Work out the finished part from the listing and answer in its coordinate system (mm). Give positions to 0.01 mm unless a question says otherwise; leave off trailing zeros. Loops run counter-clockwise (first coordinate to the right, second up) from the corner with the lowest first, then second, coordinate; pieces in that order, holes last. Notation, with made-up numbers: (62, 70) - (89, 70) arc R15 cw to (89, 94) - close; hole circle Ø2 at (-7, 31). An arc over 180 degrees is marked (long way). Use CSV: the item, a comma, the result in double quotes.
from build123d import *

# Parameters (mm, degrees)
F0_W     = 30
F0_H     = 34
F0_R     = 1.5
F1_DEPTH = 22
F2_R     = 3.95
F3_DEPTH = 32.7


with BuildPart() as f1:
    # F0 (on Top) → F1 (new body)
    with BuildSketch(Plane.XY):
        with Locations((-15, 17)):
            Rectangle(F0_W, F0_H)
        with Locations((-24, 5)):
            Circle(F0_R, mode=Mode.SUBTRACT)
        with Locations((-6, 5)):
            Circle(F0_R, mode=Mode.SUBTRACT)
        with Locations((-24, 29)):
            Circle(F0_R, mode=Mode.SUBTRACT)
        with Locations((-6, 29)):
            Circle(F0_R, mode=Mode.SUBTRACT)
    extrude(amount=F1_DEPTH)

    # F2 (on face) → F3 (cut)
    with BuildSketch(Plane.YZ):
        with Locations((17, 11)):
            Circle(F2_R)
    extrude(amount=-F3_DEPTH, mode=Mode.SUBTRACT)


solid = f1.part
Item 1: A cutting plane is placed at B-B on x = -24. Determine the outline of the cut face in (y, z).
Determined:
outline,"(0, 0) - (3.5, 0) - (3.5, 22) - (0, 22) - close; (6.5, 0) - (27.5, 0) - (27.5, 22) - (6.5, 22) - close; (30.5, 0) - (34, 0) - (34, 22) - (30.5, 22) - close; hole circle Ø7.9 at (17, 11)"
Item 2: Given P1, Ø6, axis at y = 21, z = 2.5, coming from the +X side, flat-ended and moving along its own axis, determine where the tip first touches the part or whether it passes through.
Determined:
P1,"stops at x = 0"
Item 3: A cutting plane is placed at C-C on y = 5. Determine the outline of the cut face in (x, z).
Determined:
outline,"(-30, 0) - (-25.5, 0) - (-25.5, 22) - (-30, 22) - close; (-22.5, 0) - (-7.5, 0) - (-7.5, 22) - (-22.5, 22) - close; (-4.5, 0) - (0, 0) - (0, 22) - (-4.5, 22) - close"
Item 4: The mould has two halves that part along Y. Classify faces 1 (the cylindrical face through (-24.195, 30.487, 10.846)), 2 (the flat face through (-30, 13, 8)), 3 (the flat face through (-15, 34, 11)): pulls with the +Y half, pulls with the -Y half, needs draft (parallel to the pull), parting line crosses it, or undercut.
Determined:
face 1,"undercut"
face 2,"needs draft"
face 3,"pulls with the +Y half"
Item 5: A cutting plane is placed at A-A on z = 11. Determine the outline of the cut face in (x, y), and give its area (3 significant figures).
Determined:
outline,"(-30, 0) - (0, 0) - (0, 13.05) - (-30, 13.05) - close; (-30, 20.95) - (0, 20.95) - (0, 34) - (-30, 34) - close; hole circle Ø3 at (-24, 5); hole circle Ø3 at (-24, 29); hole circle Ø3 at (-6, 5); hole circle Ø3 at (-6, 29)"
area,"755 mm²"
Item 6: Find the intervals of material crossed by line 1 (Y direction, x = -6, z = 12); line 2 (Y direction, x = -18.5, z = 13.5); line 3 (Z direction, x = -19.75, y = 17), in increasing order.
Determined:
line 1,"y = 0 to 3.5, 6.5 to 13.18, 20.82 to 27.5, 30.5 to 34"
line 2,"y = 0 to 13.94, 20.06 to 34"
line 3,"z = 0 to 7.05, 14.95 to 22"
Item 7: A cutting plane is placed at D-D on y = 17. Determine the outline of the cut face in (x, z).
Determined:
outline,"(-30, 0) - (0, 0) - (0, 7.05) - (-30, 7.05) - close; (-30, 14.95) - (0, 14.95) - (0, 22) - (-30, 22) - close"
